```python
from build123d import *

# Parameters (mm, degrees)
M5X0_8_TAPPED_HOLE1_D = 4.2
CIRPATTERN1_COUNT     = 4
SKETCH6_W             = 2.1
SKETCH6_H             = 20
CIRPATTERN2_COUNT     = 2
CIRPATTERN2_ANGLE     = 90
CHAMFER1_SIZE         = 1


with BuildPart() as part:
    # Sketch1 → Revolve1 (revolve)
    with BuildSketch(Plane.XY):
        Polygon((0, 4.1), (0, 10), (15, 10), (15, 20), (25, 20), (25, 4.1), align=None)
    revolve(axis=Axis((0, 0, 0), (1, 0, 0)))

    # M5x0.8 Tapped Hole1 (through all)
    with Locations(Plane(origin=(25, 0, 0), x_dir=(0, 0, -1), z_dir=(1, 0, 0))):
        with Locations((-14.5, 0)):
            m5x0_8_tapped_hole1 = Hole(M5X0_8_TAPPED_HOLE1_D / 2)

    # CirPattern1: M5x0.8 Tapped Hole1 ×4 about axis
    cirpattern1_axis = Axis((0, 0, 0), (1, 0, 0))
    for i in range(1, CIRPATTERN1_COUNT):
        add(m5x0_8_tapped_hole1.rotate(cirpattern1_axis, i * 360 / CIRPATTERN1_COUNT), mode=Mode.SUBTRACT)

    # Sketch6 → M5x0.8 Tapped Hole2 (revolve, cut)
    with BuildSketch(Plane(origin=(7.5, 0, 0), x_dir=(0, 0, -1), z_dir=(1, 0, 0))):
        with Locations((1.05, 10)):
            Rectangle(SKETCH6_W, SKETCH6_H)
    m5x0_8_tapped_hole2 = revolve(axis=Axis((7.5, -6.35, 0), (0, 1, 0)), mode=Mode.SUBTRACT)

    # CirPattern2: M5x0.8 Tapped Hole2 ×2 about axis
    cirpattern2_axis = Axis((25, 0, 0), (-1, 0, 0))
    for i in range(1, CIRPATTERN2_COUNT):
        add(m5x0_8_tapped_hole2.rotate(cirpattern2_axis, i * CIRPATTERN2_ANGLE / (CIRPATTERN2_COUNT - 1)), mode=Mode.SUBTRACT)

    # Chamfer1
    chamfer1_edges = [part.edges().sort_by_distance(p)[0] for p in [
        (25, -4.1, 0),
        (25, -20, 0),
        (15, -20, 0),
        (0, -10, 0),
        (0, -4.1, 0),
    ]]
    chamfer(chamfer1_edges, length=CHAMFER1_SIZE)


solid = part.part
```
Can you work these out from the model? Positions are in its coordinate system, mm. A direction names the side the tool comes from. Round coordinates to 2 decimals unless told otherwise and drop trailing zeros. Loops run counter-clockwise (first coordinate to the right, second up) from the corner with the lowest first, then second, coordinate; pieces in that order, holes last. Notation, with made-up numbers: (81.5, 70) -> (128.5, 70) arc R26 ccw to (128.5, 106) -> close; hole circle Ø1 at (65, 63.5). An arc over 180 degrees is marked (long way). One line per item, written item: value. Start each with the question number.
1. If we section it at D-D, the plane x = 3: Write out the boundary of the cut face in (y, z), then the cut area to 3 significant figures.
2. If I drill on probe 1 along Z at (x, y) = (4, 0); probe 2 along X at (y, z) = (12, -9); probe 3 along Z at (x, y) = (18, 14.5), over which ranges is the centre line in solid material (lowest first)?
3. If we section it at A-A, the plane y = 0: Give the number of separate pieces and of enclosed holes in the cut face, then the cut area to 3 significant figures.
4. For faces 1 (the cylindrical face through (7.41, 6.81, 2.1)), 2 (the flat face through (15, -8, -8)), 3 (the cylindrical face through (19.93, -0.09, -12.4)), which set-ups out of +Z, -Z, +X, -X, +Y, -Y let a thin tool reach every point of the face, with its end or its side?
5. If we section it at C-C, the plane x = 18: Write out the boundary of the cut face in (y, z).
6. If we mould it in two halves opening along Z, with no side actions, what happens to faces 4 (the cylindrical face through (8.1, -2.17, -9.76)), 5 (the cylindrical face through (19.93, -12.4, 0.09)), 6 (the cylindrical face through (7.41, 2.1, -6.81))? For each: pulls with the +Z half, pulls with the -Z half, needs draft (parallel to the pull), parting line crosses it, or undercut.
7. If we section it at B-B, the plane x = 7.5: Write out the boundary of the cut face in (y, z).
8. For pin 1 (5.5 mm diameter, centred on x = 7.5, y = 0, fed in from +Z); pin 2 (1 mm diameter, centred on y = -10, z = -6, fed in from -X); pin 3 (3.5 mm diameter, centred on x = 7.5, z = 0, fed in from +Y), each with a flat end and sliding along its axis, tell me the tip position at first contact or that it passes through.
Calculated:
1. outline: circle Ø20 at (0, 0); hole circle Ø8.2 at (0, 0)
1. area: 261 mm²
2. probe 1: z = -10 to -4.1, 4.1 to 10
2. probe 2: x = 15 to 25
2. probe 3: z = -13.77 to -2.1, 2.1 to 13.77
3. separate pieces: 5
3. enclosed holes: 0
3. area: 381 mm²
4. face 1: +Y
4. face 2: -X
4. face 3: +X, -X
5. outline: circle Ø40 at (0, 0); hole circle Ø4.2 at (-14.5, 0); hole circle Ø8.2 at (0, 0); hole circle Ø4.2 at (0, -14.5); hole circle Ø4.2 at (0, 14.5); hole circle Ø4.2 at (14.5, 0)
6. face 4: parting line crosses it
6. face 5: undercut
6. face 6: needs draft
7. outline: (-2.1, -9.78) -> (-2.1, -3.52) arc R4.1 cw (long way) to (3.52, 2.1) -> (9.78, 2.1) arc R10 ccw (long way) to start; (2.1, -9.78) arc R10 ccw to (9.78, -2.1) -> (3.52, -2.1) arc R4.1 cw to (2.1, -3.52) -> close
8. pin 1: stops at z = 10
8. pin 2: stops at x = 15
8. pin 3: stops at y = -3.71
